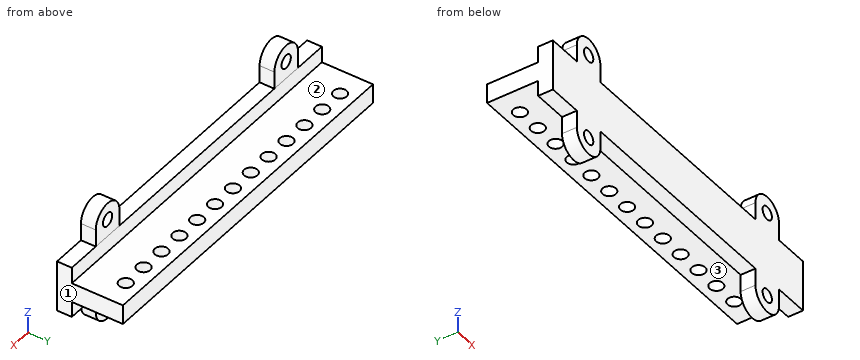
from build123d import *

# Parameters (mm, degrees)
SKETCH1_W           = 88.9
SKETCH1_H           = 25.4
BOSS_EXTRUDE1_DEPTH = 4.826
SKETCH3_W           = 88.9
SKETCH3_H           = 12.7
CUT_EXTRUDE2_DEPTH  = 93.583261317
BOSS_EXTRUDE2_DEPTH = 88.9
SKETCH7_W           = 88.9
SKETCH7_H           = 2.676927262
CUT_EXTRUDE3_DEPTH  = 94.331081232
SKETCH9_W           = 4.826
SKETCH9_H           = 6.35
BOSS_EXTRUDE3_DEPTH = 88.9
SKETCH11_R          = 1.651
CUT_EXTRUDE4_DEPTH  = 95.800625252
SKETCH13_R          = 1.651
BOSS_EXTRUDE4_DEPTH = 3.683


with BuildPart() as part:
    # Sketch1 → Boss-Extrude1 (new body)
    with BuildSketch(Plane.XY):
        with Locations((-44.45, 12.7)):
            Rectangle(SKETCH1_W, SKETCH1_H)
    extrude(amount=BOSS_EXTRUDE1_DEPTH)

    # Sketch3 → Cut-Extrude2 (cut, through all)
    with BuildSketch(Plane.XY.offset(4.826)):
        with Locations((-44.45, 6.35)):
            Rectangle(SKETCH3_W, SKETCH3_H)
    extrude(amount=-CUT_EXTRUDE2_DEPTH, mode=Mode.SUBTRACT)

    # Sketch6 → Boss-Extrude2 (add)
    with BuildSketch(Plane.ZY.offset(88.9)):
        Polygon((2.413, 12.7), (8.855255209, 12.7), (8.855255209, 19.05), (-3.885259846, 19.05), (-3.885259846, 12.7), align=None)
    extrude(amount=-BOSS_EXTRUDE2_DEPTH)

    # Sketch7 → Cut-Extrude3 (cut, through all)
    with BuildSketch(Plane.XY.offset(8.855255209)):
        with Locations((-44.45, 14.038463631)):
            Rectangle(SKETCH7_W, SKETCH7_H)
    extrude(amount=-CUT_EXTRUDE3_DEPTH, mode=Mode.SUBTRACT)

    # Sketch9 → Boss-Extrude3 (add)
    with BuildSketch(Plane.ZY.offset(88.9)):
        with Locations((2.413, 28.575)):
            Rectangle(SKETCH9_W, SKETCH9_H)
    extrude(amount=-BOSS_EXTRUDE3_DEPTH)

    # Sketch11 → Cut-Extrude4 (cut, through all)
    with BuildSketch(Plane.XY.offset(4.826)):
        with Locations((-82.557217843, 28.012581488)):
            Circle(SKETCH11_R)
        with Locations((-76.207217843, 28.012581488)):
            Circle(SKETCH11_R)
        with Locations((-69.857217843, 28.012581488)):
            Circle(SKETCH11_R)
        with Locations((-63.507217843, 28.012581488)):
            Circle(SKETCH11_R)
        with Locations((-57.157217843, 28.012581488)):
            Circle(SKETCH11_R)
        with Locations((-50.807217843, 28.012581488)):
            Circle(SKETCH11_R)
        with Locations((-44.457217843, 28.012581488)):
            Circle(SKETCH11_R)
        with Locations((-38.107217843, 28.012581488)):
            Circle(SKETCH11_R)
        with Locations((-31.757217843, 28.012581488)):
            Circle(SKETCH11_R)
        with Locations((-25.407217843, 28.012581488)):
            Circle(SKETCH11_R)
        with Locations((-19.057217843, 28.012581488)):
            Circle(SKETCH11_R)
        with Locations((-12.707217843, 28.012581488)):
            Circle(SKETCH11_R)
        with Locations((-6.357217843, 28.012581488)):
            Circle(SKETCH11_R)
    extrude(amount=-CUT_EXTRUDE4_DEPTH, mode=Mode.SUBTRACT)

    # Sketch13 → Boss-Extrude4 (add)
    # profile 1 of 2: a face of its own
    with BuildSketch(Plane(origin=(0, 15.376927262, 0), x_dir=(-1, 0, 0), z_dir=(0, -1, 0))):
        with BuildLine():
            Line((80.391, -8.855255209), (80.391, -13.173255209))
            ThreePointArc((80.391, -13.173255209), (76.2, -17.364255209), (72.009, -13.173255209))
            Line((72.009, -13.173255209), (72.009, -8.855255209))
            Line((72.009, -8.855255209), (80.391, -8.855255209))
        make_face()
        with Locations(Location((76.2, -13.173255209, 0), (0, 0, 90))):
            Circle(SKETCH13_R, mode=Mode.SUBTRACT)
    # profile 2 of 2: a face of its own
    with BuildSketch(Plane(origin=(0, 15.376927262, 0), x_dir=(-1, 0, 0), z_dir=(0, -1, 0))):
        with BuildLine():
            Line((72.009, 3.885259846), (72.009, 8.203259846))
            ThreePointArc((72.009, 8.203259846), (76.2, 12.394259846), (80.391, 8.203259846))
            Line((80.391, 8.203259846), (80.391, 3.885259846))
            Line((80.391, 3.885259846), (72.009, 3.885259846))
        make_face()
        with Locations(Location((76.2, 8.203259846, 0), (0, 0, 90))):
            Circle(SKETCH13_R, mode=Mode.SUBTRACT)
    boss_extrude4 = extrude(amount=-BOSS_EXTRUDE4_DEPTH)

    # Mirror2: Boss-Extrude4 across plane
    add(boss_extrude4.mirror(Plane(origin=(-44.45, 0, 0), x_dir=(0, 0, 1), z_dir=(1, 0, 0))))


solid = part.part
Geometry check sheet. Reference: the model listing, model coordinates, mm. Face numbers are marked on the shaded views. A direction names the side the tool comes from. Round coordinates to 2 decimals unless told otherwise and drop trailing zeros. Order: outer loops, then holes, each group sorted by start corner. A loop starts at its lowest first (then second) coordinate and runs counter-clockwise, first axis right, second up. Notation, with made-up numbers: M 47.5,81 L 52.5,81 A22 ccw 52.5,98 Z; hole C 78.5,25.5 d4. An arc over 180 degrees is marked long. Answer in a Markdown table with one row per item. Add a question column.
Item 1: Material ranges on L1, parallel to Z at x = -85, y = 25; L2, parallel to Y at x = -10.5, z = 12.5; L3, parallel to Y at x = -20, z = 1.25, recorded low to high. Write a range as [from, to].
Item 2: Sectioned sample at D-D, the plane y = 23. Enter the section's corners in (x, z).
Item 3: Set-up check for the marked faces 1, 2 and 3: record each of +Z, -Z, +X, -X, +Y, -Y from which the full face is reachable in a straight line by a thin tool's end or side.
Item 4: Depth check by flat-ended pin: pin 1 Ø4.5 at (x, y) = (-69.86, 28.01) entering from -Z; pin 2 Ø4 at (y, z) = (18, 11) entering from +X; pin 3 Ø1.1 at (x, y) = (-46.5, 17) entering from -Z. Enter the tip coordinate at first touch or a pass-through.
Item 5: Sectioned sample at B-B, the plane x = -76.2. State how many separate pieces and enclosed holes the cut face has, plus the area to 3 significant figures.
Item 6: Sectioned sample at A-A, the plane z = -5. Enter the section's corners in (x, y).
Item 7: Sectioned sample at C-C, the plane x = -47. Enter the section's corners in (y, z), plus the area to 3 significant figures.
Filled in:
| question | item | result |
|---|---|---|
| 1 | L1 | z = [0, 4.83] |
| 1 | L2 | y = [15.38, 19.06] |
| 1 | L3 | y = [15.38, 26.66], [29.37, 31.75] |
| 2 | outline | M -88.9,0 L 0,0 L 0,4.83 L -88.9,4.83 Z |
| 3 | face 1 | +Z, -Z, +X, +Y, -Y |
| 3 | face 2 | +Z, +X, -X, +Y |
| 3 | face 3 | -Z, +X, -X, +Y |
| 4 | pin 1 | stops at z = 0 |
| 4 | pin 2 | stops at x = -8.51 |
| 4 | pin 3 | stops at z = -3.89 |
| 5 | separate pieces | 4 |
| 5 | enclosed holes | 0 |
| 5 | area | 131 mm² |
| 6 | outline | M -80.39,15.38 L -72.01,15.38 L -72.01,19.06 L -80.39,19.06 Z; M -16.89,15.38 L -8.51,15.38 L -8.51,19.06 L -16.89,19.06 Z |
| 7 | outline | M 15.38,-3.89 L 19.05,-3.89 L 19.05,0 L 31.75,0 L 31.75,4.83 L 19.05,4.83 L 19.05,8.86 L 15.38,8.86 Z |
| 7 | area | 108 mm² |
